```python
from build123d import *

# Parameters (mm, degrees)
PAD_DEPTH    = 5
SKETCH001_R  = 1.75
POCKET_DEPTH = 3.001
CHAMFER_SIZE = 1.8


with BuildPart() as part:
    # Sketch → Pad (new body, symmetric)
    with BuildSketch(Plane.YZ):
        Polygon((-11.25, 3), (11.25, 3), (11.25, -1.196), (14, -1.196), (14, 3), (16.5, 3), (16.5, -4.196), (11.696, -4.196), (7.5, 0), (-7.5, 0), (-11.696, -4.196), (-16.5, -4.196), (-16.5, 3), (-14, 3), (-14, -1.196), (-11.25, -1.196), align=None)
    extrude(amount=PAD_DEPTH, both=True)

    # Sketch001 → Pocket (cut, through all)
    with BuildSketch(Plane.XY):
        with Locations((0, 3)):
            Circle(SKETCH001_R)
    extrude(amount=POCKET_DEPTH, mode=Mode.SUBTRACT)

    # Chamfer
    chamfer_edges = [part.edges().sort_by_distance(p)[0] for p in [
        (-1.75, 3, 0),
    ]]
    chamfer(chamfer_edges, length=CHAMFER_SIZE)


solid = part.part
```
Here's how the part is built. I have some questions about the finished solid (model axes, mm). A direction names the side the tool comes from. Give positions to 0.01 mm unless a question says otherwise; leave off trailing zeros. Write each loop counter-clockwise with the first axis right and the second up, starting at its lowest first coordinate (ties: lowest second). Pieces come first, ordered by that corner, then holes. Notation, with made-up numbers: M 51.25,35.25 L 108.25,35.25 A27 cw 108.25,65.25 Z; hole C 42,-21.5 d6. An arc over 180 degrees is marked long. Put each result on its own line as item: value. Start each with the question number.
Item 1: If we section it at B-B, the plane y = 3: Write out the boundary of the cut face in (x, z), then the cut area to 3 significant figures.
Item 2: If we section it at D-D, the plane x = 0: Write out the boundary of the cut face in (y, z), then the cut area to 3 significant figures.
Item 3: I need wall thicknesses on L1, parallel to Y at x = 0, z = 2.15; L2, parallel to Y at x = -2.5, z = 1.75; L3, parallel to X at y = 3, z = 2.2. Which ranges of each line are inside material? Lowest first, please. Write a range as from..to.
Item 4: On a 3-axis mill with a long thin cutter (end or side, diameter ignored), from which of +Z, -Z, +X, -X, +Y, -Y can I reach the whole of each face in a straight line? I mean faces 1 (the flat face through (0, -14, -4.196)), 2 (the flat face through (0.1, 9.6, -2.1)), 3 (the flat face through (0, 14, 1)). Say none if no direction works.
Item 5: Thinking about a two-plate mould opening in X: for faces 4 (the flat face through (-5, 0.2, 0.3)), 5 (the conical face through (-0.242, 4.847, 1.687)), 6 (the flat face through (0, 13, -1.196)), which applies, +X half, -X half, draft (parallel to the pull), parting line (faces both ways), or undercut?
Item 6: If we section it at A-A, the plane z = -2.5: Write out the boundary of the cut face in (x, y), then the cut area to 3 significant figures.
Item 7: Will these pins go through, and if not, where does the flat tip stop? pin 1 (2 mm diameter, centred on x = -1, y = 12.5, fed in from +Z); pin 2 (5.5 mm diameter, centred on x = 0, y = 3, fed in from -Z); pin 3 (4 mm diameter, centred on x = 3, y = 10.5, fed in from -Z).
Item 8: If we section it at C-C, the plane z = 2.5: Write out the boundary of the cut face in (x, y), then the cut area to 3 significant figures.
Values:
1. outline: M -5,0 L -3.55,0 L -1.75,1.8 L -1.75,3 L -5,3 Z; M 1.75,1.8 L 3.55,0 L 5,0 L 5,3 L 1.75,3 Z
1. area: 16.3 mm²
2. outline: M -16.5,-4.2 L -11.7,-4.2 L -7.5,0 L -0.55,0 L 1.25,1.8 L 1.25,3 L -11.25,3 L -11.25,-1.2 L -14,-1.2 L -14,3 L -16.5,3 Z; M 4.75,1.8 L 6.55,0 L 7.5,0 L 11.7,-4.2 L 16.5,-4.2 L 16.5,3 L 14,3 L 14,-1.2 L 11.25,-1.2 L 11.25,3 L 4.75,3 Z
2. area: 120 mm²
3. L1: -16.5..-14, -11.25..1.25, 4.75..11.25, 14..16.5
3. L2: -16.5..-14, -11.25..11.25, 14..16.5
3. L3: -5..-1.75, 1.75..5
4. face 1: -Z, +X, -X, +Y, -Y
4. face 2: -Z, +X, -X
4. face 3: +Z, +X, -X
5. face 4: -X half
5. face 5: undercut
5. face 6: draft
6. outline: M -5,-16.5 L 5,-16.5 L 5,-10 L -5,-10 Z; M -5,10 L 5,10 L 5,16.5 L -5,16.5 Z
6. area: 130 mm²
7. pin 1: z = -1.2
7. pin 2: z = 0.8
7. pin 3: z = -4.2
8. outline: M -5,-16.5 L 5,-16.5 L 5,-14 L -5,-14 Z; M -5,-11.25 L 5,-11.25 L 5,11.25 L -5,11.25 Z; M -5,14 L 5,14 L 5,16.5 L -5,16.5 Z; hole C 0,3 d3.5
8. area: 265 mm²
